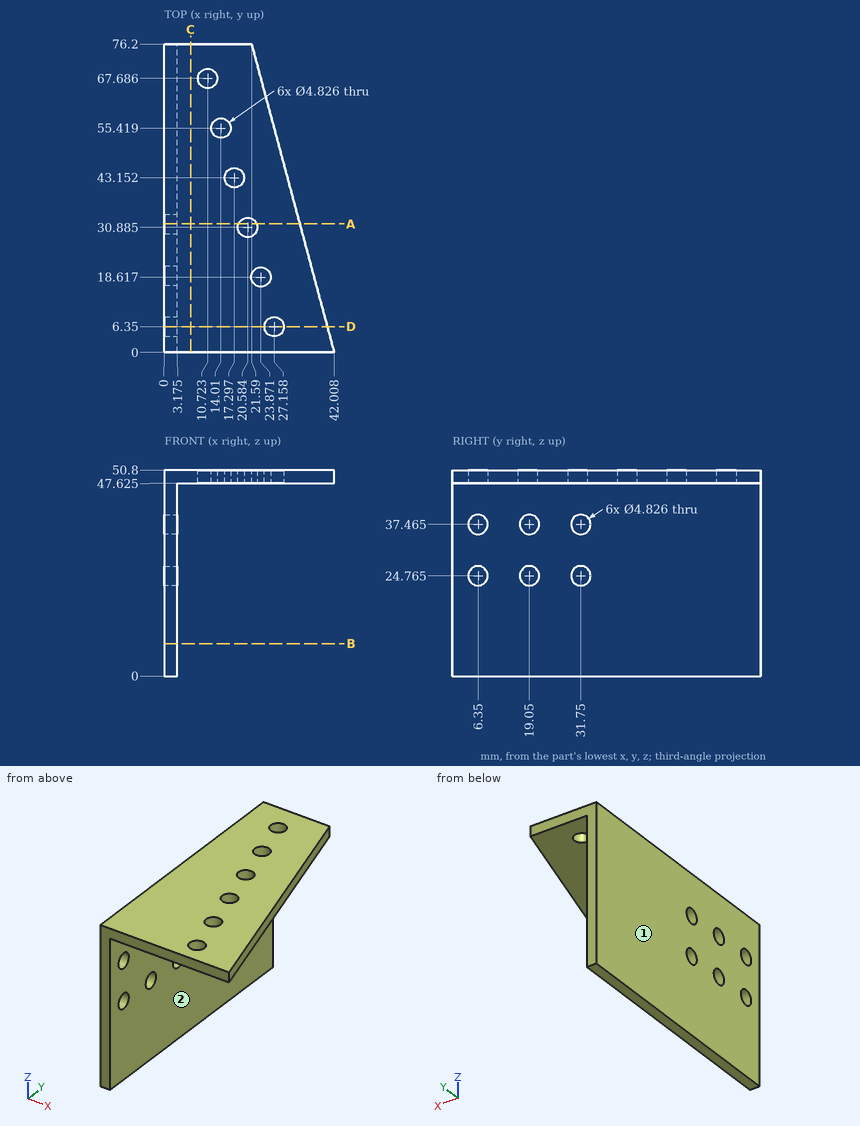
Geometry: see drawing. Coordinates: mm, zero at the bounding-box minimum. A direction names the side the tool comes from. Coordinates: 2 decimals unless noted, no trailing zeros. Loops run counter-clockwise (first coordinate to the right, second up) from the corner with the lowest first, then second, coordinate; pieces in that order, holes last. Notation, with made-up numbers: (34.5, 0) - (57.5, 0) arc R26 ccw to (57.5, 16) - close; hole circle Ø3 at (-35, 7). An arc over 180 degrees is marked (long way). Answer in a Markdown table with one row per item.
(1) Cut plane A-A on y = 31.75. Output: boundary loops of the cut face in (x, z) (1 decimal).
Model answer:
| item | result |
|---|---|
| outline | (0, 0) - (3.2, 0) - (3.2, 22.4) - (0, 22.4) - close; (0, 27.2) - (3.2, 27.2) - (3.2, 35.1) - (0, 35.1) - close; (0, 39.9) - (3.2, 39.9) - (3.2, 47.6) - (18.3, 47.6) - (18.3, 50.8) - (0, 50.8) - close; (22.8, 47.6) - (33.5, 47.6) - (33.5, 50.8) - (22.8, 50.8) - close |
(2) Cut plane B-B on z = 8. Output: boundary loops of the cut face in (x, y) (1 decimal).
Model answer:
| item | result |
|---|---|
| outline | (0, 0) - (3.2, 0) - (3.2, 76.2) - (0, 76.2) - close |
(3) Pin query (flat end, axial travel): P1, Ø7.5, axis at y = 19.05, z = 37.465, coming from the +X side (1 decimal); P2, Ø3, axis at y = 19.05, z = 24.765, coming from the +X side (3 decimals); P3, Ø8, axis at x = 20.5, y = 37, coming from the -Z side (1 decimal). Return the tip coordinate at first contact, or that it passes through.
Model answer:
| item | result |
|---|---|
| P1 | stops at x = 3.2 |
| P2 | passes through |
| P3 | stops at z = 47.6 |
(4) Cut plane D-D on y = 6.35. Output: boundary loops of the cut face in (x, z) (1 decimal), plus the area to 3 significant figures.
Model answer:
| item | result |
|---|---|
| outline | (0, 0) - (3.2, 0) - (3.2, 22.4) - (0, 22.4) - close; (0, 27.2) - (3.2, 27.2) - (3.2, 35.1) - (0, 35.1) - close; (0, 39.9) - (3.2, 39.9) - (3.2, 47.6) - (24.7, 47.6) - (24.7, 50.8) - (0, 50.8) - close; (29.6, 47.6) - (40.3, 47.6) - (40.3, 50.8) - (29.6, 50.8) - close |
| area | 233 mm² |
(5) Set-up query: the marked faces 1 and 2. Return all of +Z, -Z, +X, -X, +Y, -Y with unobstructed straight access to the full face (end or side cutting, diameter ignored); none if empty.
Model answer:
| item | result |
|---|---|
| face 1 | +Z, -Z, -X, +Y, -Y |
| face 2 | -Z, +X, +Y, -Y |
(6) Material intervals for L1, parallel to Z at x = 1, y = 19; L2, parallel to X at y = 9.5, z = 5 (1 decimal); L3, parallel to Z at x = 22, y = 55 (1 decimal), sorted ascending. Write a range as from..to.
Model answer:
| item | result |
|---|---|
| L1 | z = 0..22.35, 27.18..35.05, 39.88..50.8 |
| L2 | x = 0..3.2 |
| L3 | z = 47.6..50.8 |
(7) Cut plane C-C on x = 6.5. Output: boundary loops of the cut face in (y, z) (1 decimal).
Model answer:
| item | result |
|---|---|
| outline | (0, 47.6) - (76.2, 47.6) - (76.2, 50.8) - (0, 50.8) - close |
